```python
from build123d import *

# Parameters (mm, degrees)
F0_R     = 6
F1_DEPTH = 2.5
F2_R     = 4
F3_DEPTH = 17
F4_R     = 2
F5_DEPTH = 10


with BuildPart() as f1:
    # F0 (on Front) → F1 (new body, symmetric)
    with BuildSketch(Plane.XZ):
        Circle(F0_R)
    extrude(amount=F1_DEPTH, both=True)

    # F2 (on face) → F3 (join)
    with BuildSketch(Plane.XZ.offset(2.5)):
        Circle(F2_R)
    extrude(amount=F3_DEPTH)

    # F4 (on face) → F5 (cut)
    with BuildSketch(Plane.XZ.offset(19.5)):
        Circle(F4_R)
    extrude(amount=-F5_DEPTH, mode=Mode.SUBTRACT)


solid = f1.part
```
Could you check a few things on this model? Use its own coordinates, in mm. A direction names the side the tool comes from. Give positions to 0.01 mm unless a question says otherwise; leave off trailing zeros. Write each loop counter-clockwise with the first axis right and the second up, starting at its lowest first coordinate (ties: lowest second). Pieces come first, ordered by that corner, then holes. Notation, with made-up numbers: (-32.5, 52) -> (-4.5, 52) arc R23 cw to (-4.5, 74) -> close; hole circle Ø4 at (61.25, -23.5). An arc over 180 degrees is marked (long way). Write each question's results on one line, items separated by ' | '.
1. I need wall thicknesses on L1, parallel to Z at x = 0, y = -17; L2, parallel to Y at x = -5.5, z = 0.5; L3, parallel to X at y = -18.5, z = -0.25. Which ranges of each line are inside material? Lowest first, please.
Check sheet entries:
L1: z = -4 to -2, 2 to 4 | L2: y = -2.5 to 2.5 | L3: x = -3.99 to -1.98, 1.98 to 3.99
2. On a 3-axis mill with a long thin cutter (end or side, diameter ignored), from which of +Z, -Z, +X, -X, +Y, -Y can I reach the whole of each face in a straight line? I mean faces 5 (the flat face through (-1.42, -2.5, -3.92)), 6 (the cylindrical face through (-6, 0, 0)). Say none if no direction works.
Check sheet entries:
face 5: -Y | face 6: +Y, -Y
3. I want a section at C-C, the plane y = -5. Write out the boundary of the cut face in (x, z).
Check sheet entries:
outline: circle Ø8 at (0, 0)
4. I want a section at A-A, the plane z = 0. Write out the boundary of the cut face in (x, y), then the cut area to 3 significant figures.
Check sheet entries:
outline: (-6, -2.5) -> (-4, -2.5) -> (-4, -19.5) -> (-2, -19.5) -> (-2, -9.5) -> (2, -9.5) -> (2, -19.5) -> (4, -19.5) -> (4, -2.5) -> (6, -2.5) -> (6, 2.5) -> (-6, 2.5) -> close | area: 156 mm²
5. Will these pins go through, and if not, where does the flat tip stop? pin 1 Ø1.5 at (x, y) = (1.5, -9.5) entering from -Z; pin 2 Ø5 at (x, y) = (0.5, -5.5) entering from +Z; pin 3 Ø2 at (y, z) = (-14, -1.5) entering from -X; pin 4 Ø4.5 at (x, z) = (0.5, 0.5) entering from -Y.
Check sheet entries:
pin 1: stops at z = -3.93 | pin 2: stops at z = 4 | pin 3: stops at x = -3.97 | pin 4: stops at y = -19.5
6. I want a section at B-B, the plane x = 0. Write out the boundary of the cut face in (y, z), then the cut area to 3 significant figures.
Check sheet entries:
outline: (-19.5, -4) -> (-2.5, -4) -> (-2.5, -6) -> (2.5, -6) -> (2.5, 6) -> (-2.5, 6) -> (-2.5, 4) -> (-19.5, 4) -> (-19.5, 2) -> (-9.5, 2) -> (-9.5, -2) -> (-19.5, -2) -> close | area: 156 mm²
7. If we mould it in two halves opening along X, with no side actions, what happens to faces 1 (the flat face through (0, 2.5, 0)), 2 (the flat face through (0, -9.5, 0)), 3 (the cylindrical face through (-0.867, -10.881, -3.905)), 4 (the cylindrical face through (0, -15, -2))? For each: released by +X, released by -X, zero draft, split by the parting line, or undercut.
Check sheet entries:
face 1: zero draft | face 2: undercut | face 3: split by the parting line | face 4: undercut
8. I want a section at D-D, the plane y = -17. Write out the boundary of the cut face in (x, z), then the cut area to 3 significant figures.
Check sheet entries:
outline: circle Ø8 at (0, 0); hole circle Ø4 at (0, 0) | area: 37.7 mm²
